Geometry check sheet. Reference: drawing and pictorial views, mm from the part's lowest x, y, z. A direction names the side the tool comes from. Round coordinates to 2 decimals unless told otherwise and drop trailing zeros. Order: outer loops, then holes, each group sorted by start corner. A loop starts at its lowest first (then second) coordinate and runs counter-clockwise, first axis right, second up.
(1) Thickness scan on probe 1 along Z at (x, y) = (4, 0.55); probe 2 along X at (y, z) = (0.5, 91); probe 3 along X at (y, z) = (0.9, 55). Record the ranges inside material, lowest first.
(2) Sectioned sample at C-C, the plane y = 8. Enter the section's corners in (x, z) (1 decimal), and give its area (3 significant figures).
(3) Tool access check on the marked faces 1, 2, 3 and 4. Record the directions out of +Z, -Z, +X, -X, +Y, -Y that give a thin tool (end or side, any length) a straight path to the whole face; none if there is none.
(4) Mould release check, pull along Z, two halves, no side actions. Record for the marked faces 5, 6, 7 and 8: released by +Z, released by -Z, zero draft, split by the parting line, or undercut.
(5) Sectioned sample at D-D, the plane x = 4. Enter the section's corners in (y, z).
(6) Sectioned sample at A-A, the plane z = 91. Enter the section's corners in (x, y).
(7) Depth check by flat-ended pin: pin 1 (2.5 mm diameter, centred on x = 32, z = 91, fed in from +Y); pin 2 (1 mm diameter, centred on y = 12, z = 58.5, fed in from -X); pin 3 (7.5 mm diameter, centred on x = 16, z = 13, fed in from -Y); pin 4 (3.5 mm diameter, centred on y = 6, z = 67, fed in from +X). Enter the tip coordinate at first touch or a pass-through.
(8) Sectioned sample at B-B, the plane x = 32. Enter the section's corners in (y, z).
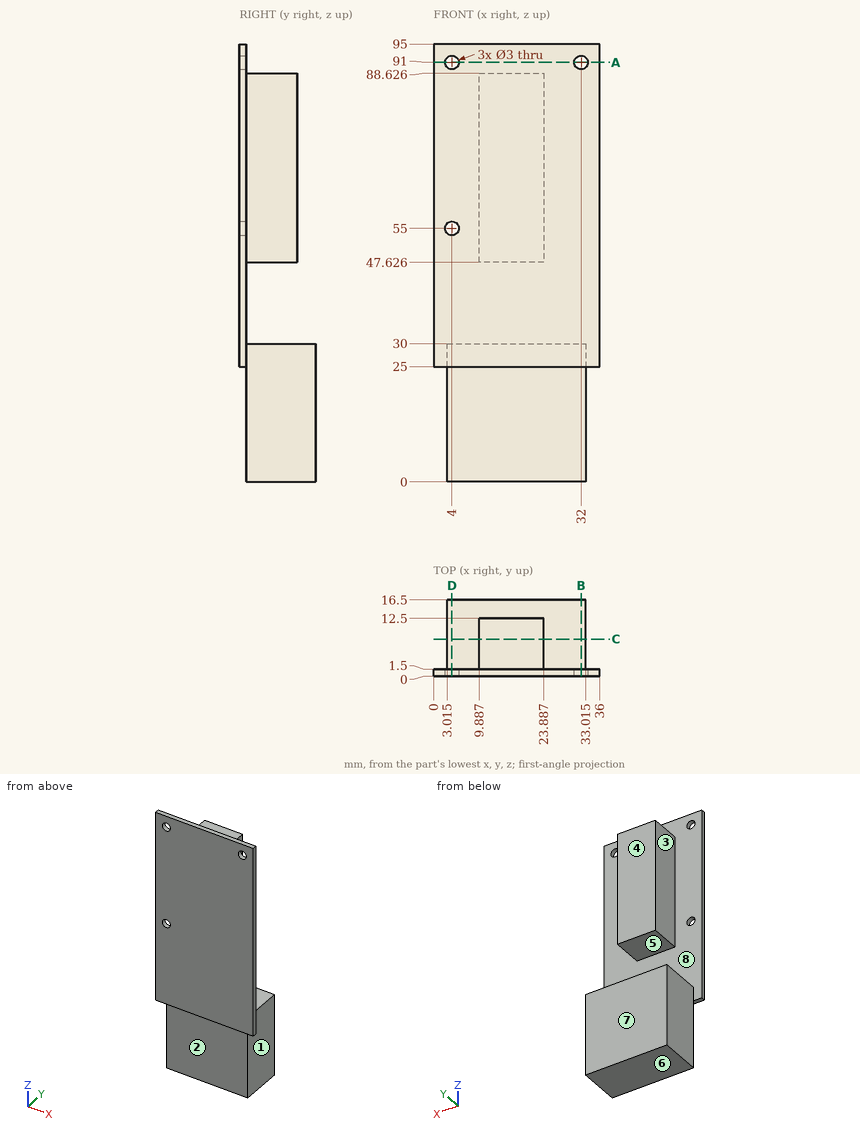
Derived:
1. probe 1: z = 25 to 53.5, 56.5 to 89.5, 92.5 to 95
1. probe 2: x = 0 to 2.5, 5.5 to 30.5, 33.5 to 36
1. probe 3: x = 0 to 2.5, 5.5 to 36
2. outline: (3, 0) - (33, 0) - (33, 30) - (3, 30) - close; (9.9, 47.6) - (23.9, 47.6) - (23.9, 88.6) - (9.9, 88.6) - close
2. area: 1,470 mm2
3. face 1: +Z, -Z, +X, +Y
3. face 2: -Z, +X, -X, -Y
3. face 3: +Z, -X, +Y
3. face 4: +Z, +X, -X, +Y
4. face 5: undercut
4. face 6: released by -Z
4. face 7: zero draft
4. face 8: undercut
5. outline: (0, 25) - (1.5, 25) - (1.5, 0) - (16.5, 0) - (16.5, 30) - (1.5, 30) - (1.5, 53.5) - (0, 53.5) - close; (0, 56.5) - (1.5, 56.5) - (1.5, 89.5) - (0, 89.5) - close; (0, 92.5) - (1.5, 92.5) - (1.5, 95) - (0, 95) - close
6. outline: (0, 0) - (2.5, 0) - (2.5, 1.5) - (0, 1.5) - close; (5.5, 0) - (30.5, 0) - (30.5, 1.5) - (5.5, 1.5) - close; (33.5, 0) - (36, 0) - (36, 1.5) - (33.5, 1.5) - close
7. pin 1: passes through
7. pin 2: stops at x = 9.89
7. pin 3: stops at y = 1.5
7. pin 4: stops at x = 23.89
8. outline: (0, 25) - (1.5, 25) - (1.5, 0) - (16.5, 0) - (16.5, 30) - (1.5, 30) - (1.5, 89.5) - (0, 89.5) - close; (0, 92.5) - (1.5, 92.5) - (1.5, 95) - (0, 95) - close
